```python
from build123d import *

# Parameters (mm, degrees)
F0_R            = 58.5548573359
F1_DEPTH        = 25.4
F2_R            = 9.9387856365
F3_DEPTH        = 25.4
F3_COPIES_COUNT = 3
F5_DEPTH        = 50.8
F5_COPIES_COUNT = 8
F6_W            = 12.9660330713
F6_H            = 12.1016278863
F7_DEPTH        = 25.4
F7_COPIES_COUNT = 8


# Not quite as in the source:
# - a pattern or mirror of a feature is missing from the dataset's text; its kind, count and spacing are read off the source's solid


with BuildPart() as f1:
    # F0 (on Top) → F1 (new body, symmetric)
    with BuildSketch(Plane.XY):
        Circle(F0_R)
    extrude(amount=F1_DEPTH, both=True)

    # F2 (on face) → F3 (join)
    with BuildSketch(Plane.XY.offset(25.4)):
        with Locations((-26.5582595021, 29.0003977716)):
            Circle(F2_R)
    f3 = extrude(amount=F3_DEPTH)

    # F3_copies: F3 ×3 about axis
    f3_copies_axis = Axis((0, 0, 0), (0, 0, 1))
    for i in range(1, F3_COPIES_COUNT):
        add(f3.rotate(f3_copies_axis, i * 360 / F3_COPIES_COUNT))

    # F4 (on face) → F5 (join, through all)
    with BuildSketch(Plane.XY.offset(25.4)):
        with BuildLine():
            Line((0, 65.528380896), (-7.4493038573, 58.0790770387))
            ThreePointArc((-7.4493038573, 58.0790770387), (0, 58.5548573359), (7.4493038573, 58.0790770387))
            Line((7.4493038573, 58.0790770387), (0, 65.528380896))
        make_face()
    f5 = extrude(amount=-F5_DEPTH)

    # F5_copies: F5 ×8 about axis
    f5_copies_axis = Axis((0, 0, 0), (0, 0, 1))
    for i in range(1, F5_COPIES_COUNT):
        add(f5.rotate(f5_copies_axis, i * 360 / F5_COPIES_COUNT))

    # F6 (on face) → F7 (cut)
    with BuildSketch(Plane.XY.offset(25.4)):
        with Locations((10.9036043286, 38.4410806)):
            Rectangle(F6_W, F6_H)
    f7 = extrude(amount=-F7_DEPTH, mode=Mode.SUBTRACT)

    # F7_copies: F7 ×8 about axis
    f7_copies_axis = Axis((0, 0, 0), (0, 0, 1))
    for i in range(1, F7_COPIES_COUNT):
        add(f7.rotate(f7_copies_axis, i * 360 / F7_COPIES_COUNT), mode=Mode.SUBTRACT)


solid = f1.part
```
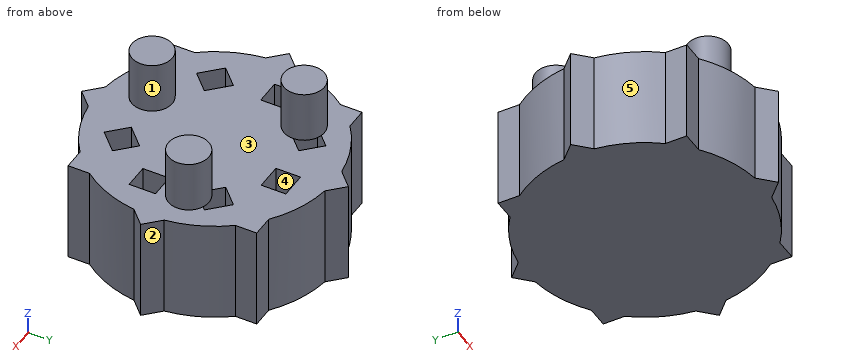
Input: part model. Units: mm. Frame: model coordinates. Face numbers are marked on the shaded views. A direction names the side the tool comes from. Round coordinates to 2 decimals unless told otherwise and drop trailing zeros. Loops run counter-clockwise (first coordinate to the right, second up) from the corner with the lowest first, then second, coordinate; pieces in that order, holes last. Notation, with made-up numbers: (27.25, 6) - (86.25, 6) arc R13 ccw to (86.25, 25) - close; hole circle Ø4 at (52.25, -7). An arc over 180 degrees is marked (long way). One line per item, written item: value. Start each with the question number.
(1) Contact query for flat-ended pins moving along their axis: P1, Ø3, axis at y = -39, z = 5.5, coming from the -X side; P2, Ø4, axis at y = 34, z = 7.5, coming from the +X side; P3, Ø10, axis at y = 4, z = -17.5, coming from the +X side. Output: stop coordinate, or through.
(2) Section B-B, the plane y = -14. Return loops of the section in (x, z).
(3) Access query for the marked faces 1 and 2. Directions: +Z, -Z, +X, -X, +Y, -Y. A direction counts if a zero-diameter tool reaches every point of the face in a straight line with its end or side. Return the directions, or none.
(4) Section A-A, the plane x = -12.5. Return loops of the section in (y, z).
(5) Section D-D, the plane x = 23. Return loops of the section in (y, z).
(6) Section C-C, the plane z = 41. Return loops of the section in (x, y).
(7) Ray query, line 1 (X direction, y = 36, z = 17); line 2 (X direction, y = -15.5, z = 8); line 3 (Z direction, x = -10.5, y = 53). Return the intervals inside material, ascending. Write a range as [from, to].
(8) Draft query along X for the marked faces 3, 4 and 5. Return one class per face: +X half, -X half, draft (parallel to the pull), parting line (faces both ways), or undercut.
Results below:
1. P1: x = -46.34
1. P2: x = 49.04
1. P3: x = 65.53
2. outline: (-56.86, -25.4) - (56.86, -25.4) - (56.86, 25.4) - (44.49, 25.4) - (44.49, 0) - (32.39, 0) - (32.39, 25.4) - (-31.81, 25.4) - (-31.81, 0) - (-38.59, 0) - (-38.59, 25.4) - (-56.86, 25.4) - close
3. face 1: +Z
3. face 2: +Z, -Z, +X, +Y
4. outline: (-57.21, -25.4) - (57.21, -25.4) - (57.21, 25.4) - (37.09, 25.4) - (37.09, 0) - (33.31, 0) - (33.31, 25.4) - (-27.58, 25.4) - (-27.58, 50.8) - (-47.42, 50.8) - (-47.42, 25.4) - (-57.21, 25.4) - close; hole (-44.49, 0) - (-32.39, 0) - (-32.39, 25.4) - (-44.49, 25.4) - close
5. outline: (-53.85, -25.4) - (53.85, -25.4) - (53.85, 25.4) - (-29.25, 25.4) - (-29.25, 0) - (-39.92, 0) - (-39.92, 25.4) - (-53.85, 25.4) - close
6. outline: circle Ø19.88 at (-26.56, 29); circle Ø19.88 at (-11.84, -37.5); circle Ø19.88 at (38.39, 8.5)
7. line 1: [-46.34, -26.92], [-11.41, 4.42], [17.39, 46.34]
7. line 2: [-56.47, -40.09], [-30.31, 32.39], [44.49, 56.47]
7. line 3: [-25.4, 25.4]
8. face 3: draft
8. face 4: undercut
8. face 5: -X half
